Geometry check sheet. Reference: drawing and pictorial views, mm from the part's lowest x, y, z. Coordinates: 2 decimals unless noted, no trailing zeros. Loops run counter-clockwise (first coordinate to the right, second up) from the corner with the lowest first, then second, coordinate; pieces in that order, holes last. Notation, with made-up numbers: (37.5, 68.5) -> (55.5, 68.5) arc R16 ccw to (55.5, 98.5) -> close; hole circle Ø4 at (-28.75, 34). An arc over 180 degrees is marked (long way). Answer as a JSON object with one key per item and string values.
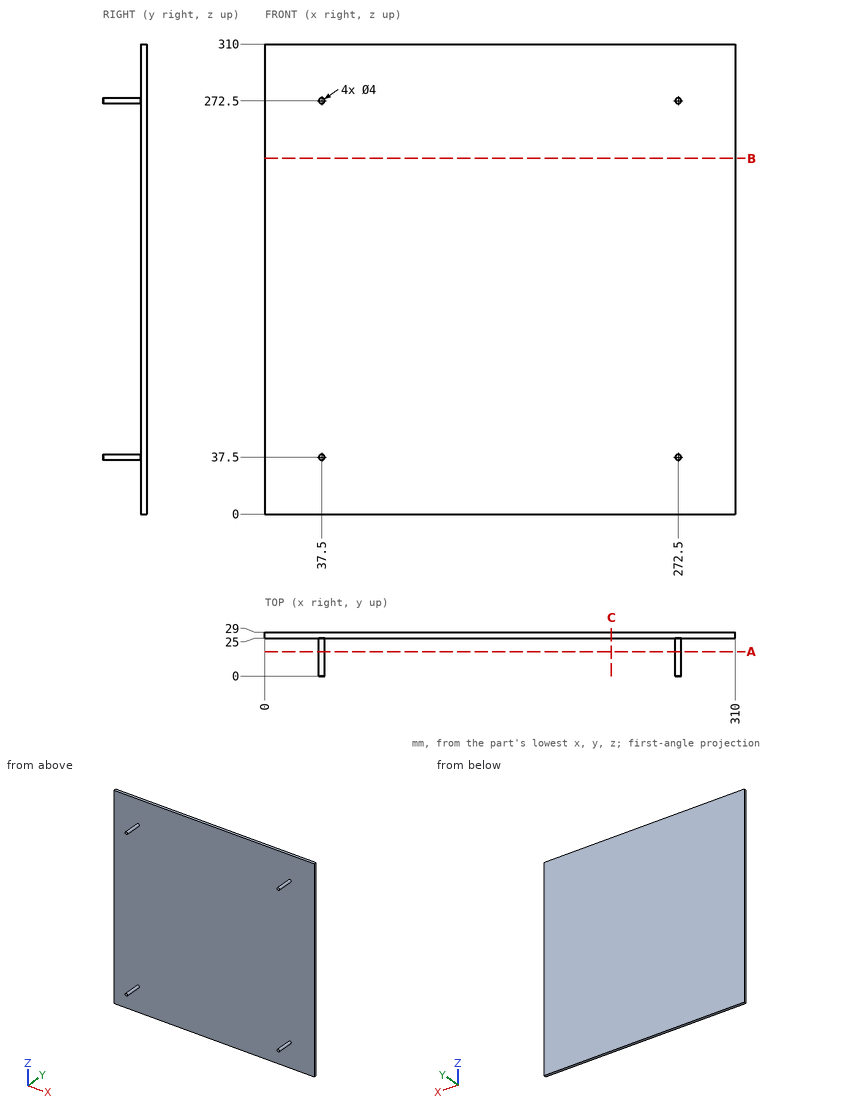
1. Thickness scan on probe 1 along Y at (x, z) = (40.5, 245.5). Record the ranges inside material, lowest first. Write a range as from..to.
Evaluation:
{"probe 1": "y = 25..29"}
2. Depth check by flat-ended pin: P1, Ø2, axis at x = 140, z = 130, coming from the -Y side; P2, Ø1, axis at y = 6, z = 268.5, coming from the -X side. Enter the tip coordinate at first touch or a pass-through.
Evaluation:
{"P1": "stops at y = 25", "P2": "passes through"}
3. Section check C-C, the plane x = 228.5. Record the boundary of the cut face in (y, z), then the cut area to 3 significant figures.
Evaluation:
{"outline": "(25, 0) -> (29, 0) -> (29, 310) -> (25, 310) -> close", "area": "1,240 mm^2"}
4. Section check B-B, the plane z = 234.5. Record the boundary of the cut face in (x, y).
Evaluation:
{"outline": "(0, 25) -> (310, 25) -> (310, 29) -> (0, 29) -> close"}
5. Section check A-A, the plane y = 16. Record the boundary of the cut face in (x, z), then the cut area to 3 significant figures.
Evaluation:
{"outline": "circle Ø4 at (37.5, 37.5); circle Ø4 at (37.5, 272.5); circle Ø4 at (272.5, 37.5); circle Ø4 at (272.5, 272.5)", "area": "50.3 mm^2"}
